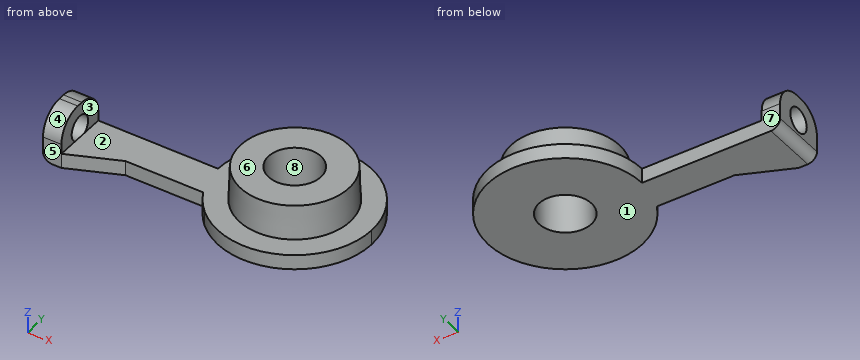
from build123d import *

# Parameters (mm, degrees)
F1_DEPTH    = 2.4
F0_W        = 3
F0_H        = 9
F2_DEPTH    = 8
F4_R        = 2
F5_DEPTH    = 3
F6_R        = 4
F7_T1_DEPTH = 16.5


# Not quite as in the source:
# - a fillet or chamfer that OpenCascade refuses, or shapes differently, is made with other operations: its cross-section is extruded or revolved along the edge and cut away or added


with BuildPart() as f1:
    # F0 (on Top) → F1 (new body)
    with BuildSketch(Plane.XY):
        with BuildLine():
            ThreePointArc((-9, 0), (-8.5094701622, -2.9306855101), (-7.0913516535, -5.5419068674))
            Line((-7.0913516535, -5.5419068674), (-4.1106286956, -5.5419068674))
            ThreePointArc((-4.1106286956, -5.5419068674), (-6.1633326212, -3.1021494161), (-6.9, 0))
            Line((-6.9, 0), (-9, 0))
        make_face()
        with BuildLine():
            ThreePointArc((-7.0913516535, -5.5419068674), (-3.9447964582, -8.0894116537), (0, -9))
            ThreePointArc((0, -9), (6.3639610307, -6.3639610307), (9, 0))
            ThreePointArc((9, 0), (0, 9), (-9, 0))
            Line((-9, 0), (-6.9, 0))
            ThreePointArc((-6.9, 0), (0, 6.9), (6.9, 0))
            ThreePointArc((6.9, 0), (3.1021494161, -6.1633326212), (-4.1106286956, -5.5419068674))
            Line((-4.1106286956, -5.5419068674), (-7.0913516535, -5.5419068674))
        make_face()
        with BuildLine():
            Line((-23.8745937477, -5.5419068674), (-11.2043414922, -5.5419068674))
            ThreePointArc((-11.2043414922, -5.5419068674), (-12.1717761369, -2.8456749066), (-12.5, 0))
            Line((-12.5, 0), (-32, 0))
            Line((-32, 0), (-32, -9))
            Line((-32, -9), (-23.8745937477, -5.5419068674))
        make_face()
        with BuildLine():
            ThreePointArc((9, 0), (6.3639610307, -6.3639610307), (0, -9))
            Line((0, -9), (-8.6746757864, -9))
            ThreePointArc((-8.6746757864, -9), (4.8896090165, -11.5039872942), (12.5, 0))
            ThreePointArc((12.5, 0), (0, 12.5), (-12.5, 0))
            Line((-12.5, 0), (-9, 0))
            ThreePointArc((-9, 0), (0, 9), (9, 0))
        make_face()
        with BuildLine():
            Line((-11.2043414922, -5.5419068674), (-7.0913516535, -5.5419068674))
            ThreePointArc((-7.0913516535, -5.5419068674), (-8.5094701622, -2.9306855101), (-9, 0))
            Line((-9, 0), (-12.5, 0))
            ThreePointArc((-12.5, 0), (-12.1717761369, -2.8456749066), (-11.2043414922, -5.5419068674))
        make_face()
        with BuildLine():
            Line((-8.6746757864, -9), (0, -9))
            ThreePointArc((0, -9), (-3.9447964582, -8.0894116537), (-7.0913516535, -5.5419068674))
            Line((-7.0913516535, -5.5419068674), (-11.2043414922, -5.5419068674))
            ThreePointArc((-11.2043414922, -5.5419068674), (-10.0887776276, -7.3801467452), (-8.6746757864, -9))
        make_face()
    extrude(amount=F1_DEPTH)

    # F0 (on Top) → F2 (join)
    with BuildSketch(Plane.XY):
        with BuildLine():
            ThreePointArc((-6.9, 0), (-6.1633326212, -3.1021494161), (-4.1106286956, -5.5419068674))
            ThreePointArc((-4.1106286956, -5.5419068674), (3.1021494161, -6.1633326212), (6.9, 0))
            ThreePointArc((6.9, 0), (0, 6.9), (-6.9, 0))
        make_face()
        with BuildLine():
            ThreePointArc((4.25, 0), (0, -4.25), (-4.25, 0))
            ThreePointArc((-4.25, 0), (0, 4.25), (4.25, 0))
        make_face(mode=Mode.SUBTRACT)
        with Locations((-33.5, -4.5)):
            Rectangle(F0_W, F0_H)
        with BuildLine():
            ThreePointArc((-7.0913516535, -5.5419068674), (-3.9447964582, -8.0894116537), (0, -9))
            ThreePointArc((0, -9), (6.3639610307, -6.3639610307), (9, 0))
            ThreePointArc((9, 0), (0, 9), (-9, 0))
            Line((-9, 0), (-6.9, 0))
            ThreePointArc((-6.9, 0), (0, 6.9), (6.9, 0))
            ThreePointArc((6.9, 0), (3.1021494161, -6.1633326212), (-4.1106286956, -5.5419068674))
            Line((-4.1106286956, -5.5419068674), (-7.0913516535, -5.5419068674))
        make_face()
        with BuildLine():
            ThreePointArc((-9, 0), (-8.5094701622, -2.9306855101), (-7.0913516535, -5.5419068674))
            Line((-7.0913516535, -5.5419068674), (-4.1106286956, -5.5419068674))
            ThreePointArc((-4.1106286956, -5.5419068674), (-6.1633326212, -3.1021494161), (-6.9, 0))
            Line((-6.9, 0), (-9, 0))
        make_face()
    extrude(amount=F2_DEPTH)

    # F4 (on offset) → F5 (cut, through all)
    with BuildSketch(Plane(origin=(-35, 0, 0), x_dir=(0, -1, 0), z_dir=(-1, 0, 0))):
        with Locations((4.5, 4)):
            Circle(F4_R)
    extrude(amount=-F5_DEPTH, mode=Mode.SUBTRACT)

    # F6
    f6_edges = [f1.edges().sort_by_distance(p)[0] for p in [
        (-33.5, -9, 8),
        (-33.5, 0, 8),
    ]]
    fillet(f6_edges, radius=F6_R)

    # F7: fillet of radius 1.5 on 2 edges, made by hand

    # F7_s2 → F7_t1 (cut)
    with BuildSketch(Plane.XZ.offset(-3.75)):
        with BuildLine():
            ThreePointArc((-35, 1.5), (-34.5606601718, 0.4393398282), (-33.5, 0))
            Line((-33.5, 0), (-35, 0))
            Line((-35, 0), (-35, 1.5))
        make_face()
    extrude(amount=F7_T1_DEPTH, mode=Mode.SUBTRACT)

    # F8: chamfer of 0.2 x 5.7272506566 on 1 edges, made by hand


with BuildPart() as f8_tool2:
    # F8_s3 → F8_t4 (revolve)
    with BuildSketch(Plane.XZ):
        Polygon((-9, 2.2727493434), (-8.8, 8), (-9, 8), align=None)
    revolve(axis=Axis((0, 0, 8), (0, 0, 1)))

    split(bisect_by=Plane.XY.offset(2.4), keep=Keep.TOP)


with BuildPart() as f1_1:
    add(f1.part)

    # F8_t1: cut F8_tool2
    add(f8_tool2.part, mode=Mode.SUBTRACT)


solid = f1_1.part
Could you check a few things on this model? Use its own coordinates, in mm. Face numbers are marked on the shaded views. A direction names the side the tool comes from. Give positions to 0.01 mm unless a question says otherwise; leave off trailing zeros. Order: outer loops, then holes, each group sorted by start corner. A loop starts at its lowest first (then second) coordinate and runs counter-clockwise, first axis right, second up.
1. For pin 1 (8 mm diameter, centred on x = -14.5, y = 1, fed in from -Z); pin 2 (0.7 mm diameter, centred on x = -16.5, z = 0.5, fed in from -Y); pin 3 (7 mm diameter, centred on x = 0, y = 0, fed in from +Z); pin 4 (4.5 mm diameter, centred on y = -5.5, z = 6.5, fed in from +X), each with a flat end and sliding along its axis, tell me the tip position at first contact or that it passes through.
Answers below:
pin 1: stops at z = 0
pin 2: stops at y = -5.54
pin 3: passes through
pin 4: stops at x = 8.24
2. Which directions (+Z, -Z, +X, -X, +Y, -Y) give clear straight access to the entire face, cutting with the end or side of a thin tool? Please do the marked faces 1, 2, 3 and 4.
Answers below:
face 1: -Z, +X, -X, +Y, -Y
face 2: +Z
face 3: +Z, +Y, -Y
face 4: +Z, -X, -Y
3. I need wall thicknesses on L1, parallel to X at y = 0.25, z = 0.75; L2, parallel to Z at x = -33, y = -4.5; L3, parallel to Z at x = -19, y = -5.25. Which ranges of each line are inside material? Lowest first, please.
Answers below:
L1: x = -12.5 to -4.24, 4.24 to 12.5
L2: z = 0 to 2, 6 to 8
L3: z = 0 to 2.4
4. Thinking about a two-plate mould opening in Y: for the marked faces 5, 6, 7 and 8, which applies, +Y half, -Y half, draft (parallel to the pull), parting line (faces both ways), or undercut?
Answers below:
face 5: -Y half
face 6: draft
face 7: +Y half
face 8: undercut
5. Suppose I cut it at D-D (y = -10.25). Write out the boundary of the cut face in (x, z).
Answers below:
outline: (-7.15, 0) - (7.15, 0) - (7.15, 2.4) - (-7.15, 2.4) - close
6. Suppose I cut it at B-B (x = 0). Write out the boundary of the cut face in (y, z).
Answers below:
outline: (-12.5, 0) - (-4.25, 0) - (-4.25, 8) - (-8.8, 8) - (-9, 2.4) - (-12.5, 2.4) - close; (4.25, 0) - (12.5, 0) - (12.5, 2.4) - (9, 2.4) - (8.8, 8) - (4.25, 8) - close
7. Suppose I cut it at A-A (z = 3). Write out the boundary of the cut face in (x, y).
Answers below:
outline: (-35, -9) - (-32, -9) - (-32, -6.23) - (-35, -6.23) - close; (-35, -2.77) - (-32, -2.77) - (-32, 0) - (-35, 0) - close; circle Ø17.95 at (0, 0); hole circle Ø8.5 at (0, 0)
8. Suppose I cut it at C-C (x = -15). Write out the boundary of the cut face in (y, z), plus the area to 3 significant figures.
Answers below:
outline: (-5.54, 0) - (0, 0) - (0, 2.4) - (-5.54, 2.4) - close
area: 13.3 mm2
